CAD build for the part. Positions are in the model's coordinates, mm. Round coordinates to 2 decimals unless told otherwise and drop trailing zeros. Loops run counter-clockwise (first coordinate to the right, second up) from the corner with the lowest first, then second, coordinate; pieces in that order, holes last. Notation, with made-up numbers: (-9, 16) - (-2, 16) arc R32 cw to (-2, 42) - close; hole circle Ø9 at (-7.5, 14.5). An arc over 180 degrees is marked (long way). One line per question, with ' | ' between items.
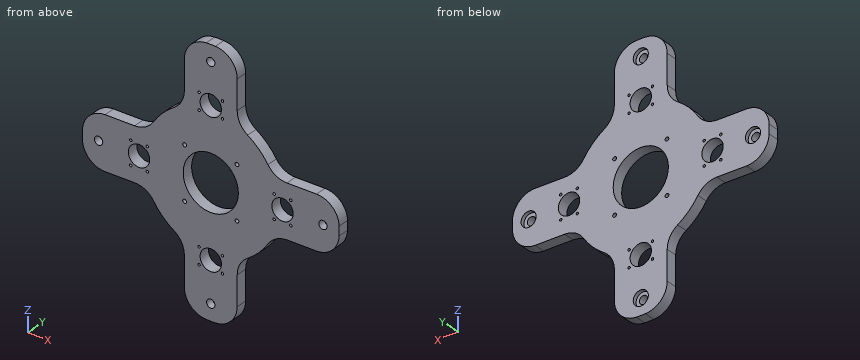
```python
from build123d import *

# Parameters (mm, degrees)
SKETCH1_R             = 36.515
BOSS_EXTRUDE1_DEPTH   = 15
FILLET1_R             = 30
M6_TAPPED_HOLE1_D     = 5
SKETCH4_R             = 10
CUT_EXTRUDE1_DEPTH    = 5
M10_CLEARANCE_HOLE1_D = 11
CIRPATTERN1_COUNT     = 4
SKETCH7_R             = 14.1
CUT_EXTRUDE2_DEPTH    = 16
CIRPATTERN2_COUNT     = 4
M4_TAPPED_HOLE1_D     = 3.3
CIRPATTERN3_COUNT     = 4


with BuildPart() as part:
    # Sketch1 → Boss-Extrude1 (new body)
    with BuildSketch(Plane(origin=(0, 0, 0), x_dir=(1, 0, 0), z_dir=(0, 1, 0))):
        with BuildLine():
            Line((-35, 166.358047596), (-35, 82.915619759))
            ThreePointArc((-35, 82.915619759), (-63.639610307, 63.639610307), (-82.915619759, 35))
            Line((-82.915619759, 35), (-166.358047596, 35))
            ThreePointArc((-166.358047596, 35), (-170, 0), (-166.358047596, -35))
            Line((-166.358047596, -35), (-82.915619759, -35))
            ThreePointArc((-82.915619759, -35), (-63.639610307, -63.639610307), (-35, -82.915619759))
            Line((-35, -82.915619759), (-35, -166.358047596))
            ThreePointArc((-35, -166.358047596), (0, -170), (35, -166.358047596))
            Line((35, -166.358047596), (35, -82.915619759))
            ThreePointArc((35, -82.915619759), (63.639610307, -63.639610307), (82.915619759, -35))
            Line((82.915619759, -35), (166.358047596, -35))
            ThreePointArc((166.358047596, -35), (170, 0), (166.358047596, 35))
            Line((166.358047596, 35), (82.915619759, 35))
            ThreePointArc((82.915619759, 35), (63.639610307, 63.639610307), (35, 82.915619759))
            Line((35, 82.915619759), (35, 166.358047596))
            ThreePointArc((35, 166.358047596), (0, 170), (-35, 166.358047596))
        make_face()
        Circle(SKETCH1_R, mode=Mode.SUBTRACT)
    extrude(amount=BOSS_EXTRUDE1_DEPTH)

    # Fillet1
    fillet1_edges = [part.edges().sort_by_distance(p)[0] for p in [
        (-166.358047596, 7.5, 35),
        (-166.358047596, 7.5, -35),
        (-82.915619759, 7.5, -35),
        (-35, 7.5, -82.915619759),
        (-35, 7.5, -166.358047596),
        (35, 7.5, -166.358047596),
        (35, 7.5, -82.915619759),
        (82.915619759, 7.5, -35),
        (166.358047596, 7.5, -35),
        (166.358047596, 7.5, 35),
        (82.915619759, 7.5, 35),
        (35, 7.5, 82.915619759),
        (35, 7.5, 166.358047596),
        (-35, 7.5, 166.358047596),
        (-35, 7.5, 82.915619759),
        (-82.915619759, 7.5, 35),
    ]]
    fillet(fillet1_edges, radius=FILLET1_R)

    # M6 Tapped Hole1 (through all)
    with Locations(Plane.XZ):
        with Locations((-34.67, -34.67), (34.67, -34.67), (34.67, 34.67), (-34.67, 34.67)):
            Hole(M6_TAPPED_HOLE1_D / 2)

    # Sketch4 → Cut-Extrude1 (cut)
    with BuildSketch(Plane(origin=(0, 15, 0), x_dir=(1, 0, 0), z_dir=(0, 1, 0))):
        with Locations((0, 148.5)):
            Circle(SKETCH4_R)
    cut_extrude1 = extrude(amount=-CUT_EXTRUDE1_DEPTH, mode=Mode.SUBTRACT)

    # M10 Clearance Hole1 (through all)
    with Locations(Plane(origin=(0, 0, 0), x_dir=(-1, 0, 0), z_dir=(0, -1, 0))):
        with Locations((0, 148.5)):
            m10_clearance_hole1 = Hole(M10_CLEARANCE_HOLE1_D / 2)

    # CirPattern1: Cut-Extrude1, M10 Clearance Hole1 ×4 about axis
    cirpattern1_axis = Axis((0, 0, 0), (0, 1, 0))
    for i in range(1, CIRPATTERN1_COUNT):
        add(cut_extrude1.rotate(cirpattern1_axis, i * 360 / CIRPATTERN1_COUNT), mode=Mode.SUBTRACT)
        add(m10_clearance_hole1.rotate(cirpattern1_axis, i * 360 / CIRPATTERN1_COUNT), mode=Mode.SUBTRACT)

    # Sketch7 → Cut-Extrude2 (cut, through all)
    with BuildSketch(Plane(origin=(0, 15, 0), x_dir=(1, 0, 0), z_dir=(0, 1, 0))):
        with Locations((0, 95)):
            Circle(SKETCH7_R)
    cut_extrude2 = extrude(amount=-CUT_EXTRUDE2_DEPTH, mode=Mode.SUBTRACT)

    # CirPattern2: Cut-Extrude2 ×4 about axis
    cirpattern2_axis = Axis((0, 0, 0), (0, 1, 0))
    for i in range(1, CIRPATTERN2_COUNT):
        add(cut_extrude2.rotate(cirpattern2_axis, i * 360 / CIRPATTERN2_COUNT), mode=Mode.SUBTRACT)

    # M4 Tapped Hole1 (through all)
    with Locations(Plane(origin=(0, 15, 0), x_dir=(1, 0, 0), z_dir=(0, 1, 0))):
        with Locations((-15.5, 106), (-15.5, 84), (15.5, 84), (15.5, 106)):
            m4_tapped_hole1 = Hole(M4_TAPPED_HOLE1_D / 2)

    # CirPattern3: M4 Tapped Hole1 ×4 about axis
    cirpattern3_axis = Axis((0, 0, 0), (0, 1, 0))
    for i in range(1, CIRPATTERN3_COUNT):
        add(m4_tapped_hole1.rotate(cirpattern3_axis, i * 360 / CIRPATTERN3_COUNT), mode=Mode.SUBTRACT)


solid = part.part
```
(1) Cut at A-A, the plane z = 148.5. Write the cut outline in (x, y), then the cut area to 3 significant figures.
Results found:
outline: (-33.74, 0) - (-5.5, 0) - (-5.5, 10) - (-10, 10) - (-10, 15) - (-33.74, 15) - close; (5.5, 0) - (33.74, 0) - (33.74, 15) - (10, 15) - (10, 10) - (5.5, 10) - close | area: 802 mm²
(2) Cut at C-C, the plane y = 3. State how many separate pieces and enclosed holes the cut face has, then the cut area to 3 significant figures.
Results found:
separate pieces: 1 | enclosed holes: 29 | area: 40,000 mm²
(3) Probe L1, parallel to Z at x = 0, y = 4.25 (3 decimals); L2, parallel to X at y = 8.25, z = 2; L3, parallel to Z at x = 106, y = 9.5. List the from-to ranges inside material, lowest first.
Results found:
L1: z = -170 to -154, -143 to -109.1, -80.9 to -36.515, 36.515 to 80.9, 109.1 to 143, 154 to 170 | L2: x = -169.99 to -153.62, -143.38 to -108.96, -81.04 to -36.46, 36.46 to 81.04, 108.96 to 143.38, 153.62 to 169.99 | L3: z = -35 to -17.15, -13.85 to -8.82, 8.82 to 13.85, 17.15 to 35
(4) Cut at D-D, the plane x = 133.5. Write the cut outline in (y, z).
Results found:
outline: (0, -35) - (15, -35) - (15, 35) - (0, 35) - close
(5) Cut at B-B, the plane x = -148.5. Write the cut outline in (y, z).
Results found:
outline: (0, -33.74) - (15, -33.74) - (15, -10) - (10, -10) - (10, -5.5) - (0, -5.5) - close; (0, 5.5) - (10, 5.5) - (10, 10) - (15, 10) - (15, 33.74) - (0, 33.74) - close
(6) Drop flat-ended pins along their axis: P1, Ø3, axis at x = 21, y = 6.5, coming from the +Z side; P2, Ø1, axis at y = 10, z = -116.5, coming from the -X side; P3, Ø4, axis at x = -30, y = 9, coming from the -Z side. Give the stop position or say it passes through.
Results found:
P1: stops at z = 166.17 | P2: stops at x = -35 | P3: stops at z = -159.17
